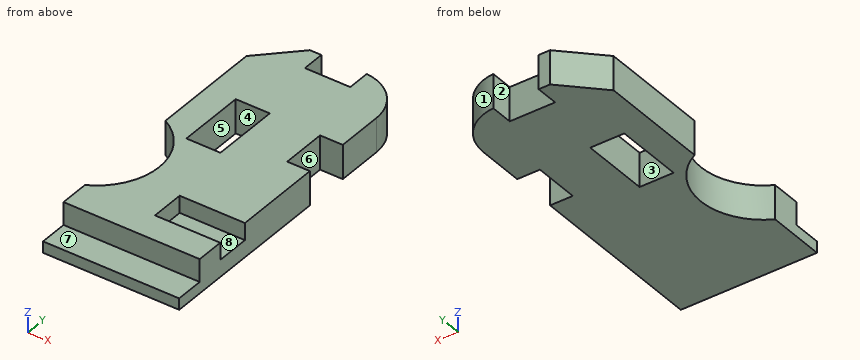
from build123d import *

# Parameters (mm, degrees)
F1_DEPTH    = 19.05
F2_W        = 76.2
F2_H        = 15.875
F3_DEPTH    = 12.7
F4_W        = 36.5125
F4_H        = 19.05
F5_DEPTH    = 9.525
F6_W        = 19.05
F6_H        = 38.1
F7_DEPTH    = 25.4
F8_T1_DEPTH = 145.8017104175


# Not quite as in the source:
# - a fillet or chamfer that OpenCascade refuses, or shapes differently, is made with other operations: its cross-section is extruded or revolved along the edge and cut away or added


with BuildPart() as f1:
    # F0 (on Top) → F1 (new body)
    with BuildSketch(Plane.XY):
        with BuildLine():
            Line((-39.025861299, -56.6028431063), (-39.025861299, -72.4778431063))
            Line((-39.025861299, -72.4778431063), (37.174138701, -72.4778431063))
            Line((37.174138701, -72.4778431063), (37.174138701, 28.547687456))
            Line((37.174138701, 28.547687456), (24.474138701, 28.547687456))
            Line((24.474138701, 28.547687456), (24.474138701, 53.947687456))
            Line((24.474138701, 53.947687456), (37.174138701, 53.947687456))
            Line((37.174138701, 53.947687456), (37.174138701, 105.3221568937))
            Line((37.174138701, 105.3221568937), (13.361638701, 105.3221568937))
            Line((13.361638701, 105.3221568937), (13.361638701, 92.6221568937))
            Line((13.361638701, 92.6221568937), (-12.038361299, 92.6221568937))
            Line((-12.038361299, 92.6221568937), (-12.038361299, 105.3221568937))
            Line((-12.038361299, 105.3221568937), (-18.388361299, 105.3221568937))
            Line((-18.388361299, 105.3221568937), (-39.025861299, 84.6846568937))
            Line((-39.025861299, 84.6846568937), (-39.025861299, 22.130676627))
            ThreePointArc((-39.025861299, 22.130676627), (-19.975861299, -8.9778431063), (-39.025861299, -40.0863628397))
            Line((-39.025861299, -40.0863628397), (-39.025861299, -40.7278431063))
            Line((-39.025861299, -40.7278431063), (-39.025861299, -56.6028431063))
        make_face()
    extrude(amount=F1_DEPTH)

    # F2 (on face) → F3 (cut)
    with BuildSketch(Plane.XY.offset(19.05)):
        with Locations((-0.925861299, -64.5403431063)):
            Rectangle(F2_W, F2_H)
    extrude(amount=-F3_DEPTH, mode=Mode.SUBTRACT)

    # F4 (on face) → F5 (cut)
    with BuildSketch(Plane.XY.offset(19.05)):
        with Locations((18.917888701, -31.2028431063)):
            Rectangle(F4_W, F4_H)
    extrude(amount=-F5_DEPTH, mode=Mode.SUBTRACT)

    # F6 (on face) → F7 (cut)
    with BuildSketch(Plane.XY.offset(19.05)):
        with Locations((-13.625861299, 35.4721568937)):
            Rectangle(F6_W, F6_H)
    extrude(amount=-F7_DEPTH, mode=Mode.SUBTRACT)

    # F8: fillet of radius 25.4 on 1 edges, made by hand

    # F8_s2 → F8_t1 (cut)
    with BuildSketch(Plane.XY.offset(-63.3758552087)):
        with BuildLine():
            ThreePointArc((37.174138701, 79.9718148102), (30.2874109671, 97.3620060109), (13.361638701, 105.3221568937))
            Line((13.361638701, 105.3221568937), (37.174138701, 105.3221568937))
            Line((37.174138701, 105.3221568937), (37.174138701, 79.9718148102))
        make_face()
    extrude(amount=F8_T1_DEPTH, mode=Mode.SUBTRACT)


solid = f1.part
Work out the finished part from the listing and answer in its coordinate system (mm). Face numbers are marked on the shaded views. A direction names the side the tool comes from. Coordinates: 2 decimals unless noted, no trailing zeros. Write each loop counter-clockwise with the first axis right and the second up, starting at its lowest first coordinate (ties: lowest second). Pieces come first, ordered by that corner, then holes.
1. Consider line 1 along Y through (x, z) = (-14.5, 5.75); line 2 along Y through (x, z) = (-14.5, 7); line 3 along X through (y, z) = (51, 5.25). Determine where each line is inside the solid, lowest interval first.
Results list:
line 1: y = -72.48 to 16.42, 54.52 to 105.32
line 2: y = -56.6 to 16.42, 54.52 to 105.32
line 3: x = -39.03 to -23.15, -4.1 to 24.47
2. Flat-ended cylindrical pins translate along their axes: pin 1 (8 mm diameter, centred on x = 15.5, y = -64, fed in from +Z); pin 2 (5 mm diameter, centred on y = -35, z = 15.5, fed in from +X); pin 3 (2 mm diameter, centred on y = 0.5, z = 14, fed in from -X). Find the tip coordinate at first contact, or state that the pin passes through.
Results list:
pin 1: stops at z = 6.35
pin 2: stops at x = 0.66
pin 3: stops at x = -21.58
3. For a pull along Y with two mould halves and no side action, classify the marked faces 1, 2, 3 and 4 as +Y half, -Y half, draft (parallel to the pull), parting line (faces both ways), or undercut.
Results list:
face 1: +Y half
face 2: draft
face 3: undercut
face 4: undercut
4. The part is cut by section D-D, the plane x = 7. Write down the section's boundary in (y, z) (3 decimals).
Results list:
outline: (-72.478, 0) - (92.622, 0) - (92.622, 19.05) - (-21.678, 19.05) - (-21.678, 9.525) - (-40.728, 9.525) - (-40.728, 19.05) - (-56.603, 19.05) - (-56.603, 6.35) - (-72.478, 6.35) - close
5. The part is cut by section A-A, the plane z = 16.5. Write down the section's boundary in (x, y) (3 decimals), and give its area (3 significant figures).
Results list:
outline: (-39.026, -56.603) - (37.174, -56.603) - (37.174, -40.728) - (0.662, -40.728) - (0.662, -21.678) - (37.174, -21.678) - (37.174, 28.548) - (24.474, 28.548) - (24.474, 53.948) - (37.174, 53.948) - (37.174, 79.972) arc R25.4 ccw to (13.362, 105.322) - (13.362, 92.622) - (-12.038, 92.622) - (-12.038, 105.322) - (-18.388, 105.322) - (-39.026, 84.685) - (-39.026, 22.131) arc R34.925 cw to (-39.026, -40.086) - close; hole (-23.151, 16.422) - (-4.101, 16.422) - (-4.101, 54.522) - (-23.151, 54.522) - close
area: 9,080 mm2
6. The part is cut by section C-C, the plane y = 43.5. Write down the section's boundary in (x, z).
Results list:
outline: (-39.03, 0) - (-23.15, 0) - (-23.15, 19.05) - (-39.03, 19.05) - close; (-4.1, 0) - (24.47, 0) - (24.47, 19.05) - (-4.1, 19.05) - close
7. The part is cut by section B-B, the plane x = -9. Write down the section's boundary in (y, z).
Results list:
outline: (-72.48, 0) - (16.42, 0) - (16.42, 19.05) - (-56.6, 19.05) - (-56.6, 6.35) - (-72.48, 6.35) - close; (54.52, 0) - (92.62, 0) - (92.62, 19.05) - (54.52, 19.05) - close
8. For the marked faces 5, 6, 7 and 8, determine the directions among +Z, -Z, +X, -X, +Y, -Y from which every point of the face is accessible in a straight line to the end or side of a thin tool.
Results list:
face 5: +Z, -Z
face 6: +Z, -Z, +X
face 7: +Z, +X, -X, -Y
face 8: +Z, +X
